from build123d import *

# Parameters (mm, degrees)
SKETCH1_W               = 393.7
SKETCH1_H               = 25.4
BOSS_EXTRUDE1_DEPTH     = 1.5875
SKETCH2_R               = 3.2639
CUT_EXTRUDE1_DEPTH      = 1
CUT_EXTRUDE1_DEPTH_BACK = 4.175


with BuildPart() as part:
    # Sketch1 → Boss-Extrude1 (new body, symmetric)
    with BuildSketch(Plane(origin=(0, 0, 0), x_dir=(1, 0, 0), z_dir=(0, 1, 0))):
        Rectangle(SKETCH1_W, SKETCH1_H)
    extrude(amount=BOSS_EXTRUDE1_DEPTH, both=True)

    # Sketch2 → Cut-Extrude1 (cut, two sides)
    with BuildSketch(Plane(origin=(0, 1.5875, 0), x_dir=(1, 0, 0), z_dir=(0, 1, 0))) as cut_extrude1_sk:
        with Locations((-184.15, 0)):
            Circle(SKETCH2_R)
        with Locations((184.15, 0)):
            Circle(SKETCH2_R)
        with Locations((-95.25, 0)):
            Circle(SKETCH2_R)
        with Locations((95.25, 0)):
            Circle(SKETCH2_R)
        with Locations((-50.8, 0)):
            Circle(SKETCH2_R)
        with Locations((50.8, 0)):
            Circle(SKETCH2_R)
    extrude(amount=CUT_EXTRUDE1_DEPTH, mode=Mode.SUBTRACT)
    extrude(cut_extrude1_sk.sketch, amount=-CUT_EXTRUDE1_DEPTH_BACK, mode=Mode.SUBTRACT)


solid = part.part
Design review of the part built by this model. Coordinates are the model's own, in mm. Give positions to 0.01 mm unless a question says otherwise; leave off trailing zeros. Order: outer loops, then holes, each group sorted by start corner. A loop starts at its lowest first (then second) coordinate and runs counter-clockwise, first axis right, second up.
1. To check wall thickness, follow L1, parallel to Z at x = -95.25, y = 0.6. State the ranges of the line that lie inside material, in increasing order.
Solution:
L1: z = -12.7 to -3.26, 3.26 to 12.7
2. Mouldability with a two-part tool opening along Z and no side actions: class faces 1 (the flat face through (-3, -1.588, 0)), 2 (the cylindrical face through (-98.51, 0.02, -0.14)) as +Z half, -Z half, draft (parallel to the pull), parting line (faces both ways), or undercut.
Solution:
face 1: draft
face 2: undercut
3. Add section A-A, the plane x = 95.25. State the section outline as (y, z) points.
Solution:
outline: (-1.59, -12.7) - (1.59, -12.7) - (1.59, -3.26) - (-1.59, -3.26) - close; (-1.59, 3.26) - (1.59, 3.26) - (1.59, 12.7) - (-1.59, 12.7) - close
4. Add section B-B, the plane z = 0. State the section outline as (x, y) points.
Solution:
outline: (-196.85, -1.59) - (-187.41, -1.59) - (-187.41, 1.59) - (-196.85, 1.59) - close; (-180.89, -1.59) - (-98.51, -1.59) - (-98.51, 1.59) - (-180.89, 1.59) - close; (-91.99, -1.59) - (-54.06, -1.59) - (-54.06, 1.59) - (-91.99, 1.59) - close; (-47.54, -1.59) - (47.54, -1.59) - (47.54, 1.59) - (-47.54, 1.59) - close; (54.06, -1.59) - (91.99, -1.59) - (91.99, 1.59) - (54.06, 1.59) - close; (98.51, -1.59) - (180.89, -1.59) - (180.89, 1.59) - (98.51, 1.59) - close; (187.41, -1.59) - (196.85, -1.59) - (196.85, 1.59) - (187.41, 1.59) - close
5. Add section C-C, the plane y = -0.95. State the section outline as (x, z) points, then the cut area to 3 significant figures.
Solution:
outline: (-196.85, -12.7) - (196.85, -12.7) - (196.85, 12.7) - (-196.85, 12.7) - close; hole circle Ø6.53 at (-184.15, 0); hole circle Ø6.53 at (-95.25, 0); hole circle Ø6.53 at (-50.8, 0); hole circle Ø6.53 at (50.8, 0); hole circle Ø6.53 at (95.25, 0); hole circle Ø6.53 at (184.15, 0)
area: 9,800 mm2
